```python
from build123d import *

# Parameters (mm, degrees)
F7_DEPTH  = 355.6
F8_D      = 12.7
F8_DEPTH  = 19.051
F9_D      = 12.7
F0_R      = 4.7625
F2_DEPTH  = 4.7625
F4_D      = 9.525
F4_DEPTH  = 19.051
F5_D      = 12.7
F5_DEPTH  = 19.051
F10_D     = 22.225
F10_DEPTH = 19.051
F6_DEPTH  = 25.4


with BuildPart() as f7:
    # F0 (on Front) → F7 (new body)
    with BuildSketch(Plane.XZ):
        with BuildLine():
            Line((-15.875, -19.05), (15.875, -19.05))
            ThreePointArc((15.875, -19.05), (18.1200640303, -18.1200640303), (19.05, -15.875))
            Line((19.05, -15.875), (19.05, 15.875))
            ThreePointArc((19.05, 15.875), (18.1200640303, 18.1200640303), (15.875, 19.05))
            Line((15.875, 19.05), (-15.875, 19.05))
            ThreePointArc((-15.875, 19.05), (-18.1200640303, 18.1200640303), (-19.05, 15.875))
            Line((-19.05, 15.875), (-19.05, -15.875))
            ThreePointArc((-19.05, -15.875), (-18.1200640303, -18.1200640303), (-15.875, -19.05))
        make_face()
        with BuildLine():
            ThreePointArc((14.2875, -11.1125), (13.3575640303, -13.3575640303), (11.1125, -14.2875))
            Line((11.1125, -14.2875), (-11.1125, -14.2875))
            ThreePointArc((-11.1125, -14.2875), (-13.3575640303, -13.3575640303), (-14.2875, -11.1125))
            Line((-14.2875, -11.1125), (-14.2875, 11.1125))
            ThreePointArc((-14.2875, 11.1125), (-13.3575640303, 13.3575640303), (-11.1125, 14.2875))
            Line((-11.1125, 14.2875), (11.1125, 14.2875))
            ThreePointArc((11.1125, 14.2875), (13.3575640303, 13.3575640303), (14.2875, 11.1125))
            Line((14.2875, 11.1125), (14.2875, -11.1125))
        make_face(mode=Mode.SUBTRACT)
    extrude(amount=F7_DEPTH)

    # F8 (through all, one way)
    with BuildSketch(Plane.XY):
        with Locations((0, -19.05)):
            Circle(F8_D / 2)
    extrude(amount=-F8_DEPTH, mode=Mode.SUBTRACT)

    # F9 (through all)
    with Locations(Plane(origin=(0, 0, 0), x_dir=(1, 0, 0), z_dir=(0, 0, -1))):
        with Locations((0, 19.05)):
            Hole(F9_D / 2)

    # F0 (on Front) → F2 (join)
    with BuildSketch(Plane.XZ):
        with BuildLine():
            Line((-11.1125, -14.2875), (11.1125, -14.2875))
            ThreePointArc((11.1125, -14.2875), (13.3575640303, -13.3575640303), (14.2875, -11.1125))
            Line((14.2875, -11.1125), (14.2875, 11.1125))
            ThreePointArc((14.2875, 11.1125), (13.3575640303, 13.3575640303), (11.1125, 14.2875))
            Line((11.1125, 14.2875), (-11.1125, 14.2875))
            ThreePointArc((-11.1125, 14.2875), (-13.3575640303, 13.3575640303), (-14.2875, 11.1125))
            Line((-14.2875, 11.1125), (-14.2875, -11.1125))
            ThreePointArc((-14.2875, -11.1125), (-13.3575640303, -13.3575640303), (-11.1125, -14.2875))
        make_face()
        Circle(F0_R, mode=Mode.SUBTRACT)
        Circle(F0_R)
    extrude(amount=F2_DEPTH)

    # F4 (through all, one way)
    with BuildSketch(Plane(origin=(0, 0, 0), x_dir=(0, 1, 0), z_dir=(-1, 0, 0))):
        with Locations((-50.8, 0)):
            Circle(F4_D / 2)
    extrude(amount=-F4_DEPTH, mode=Mode.SUBTRACT)

    # F5 (through all, one way)
    with BuildSketch(Plane.YZ):
        with Locations((-50.8, 0)):
            Circle(F5_D / 2)
    extrude(amount=-F5_DEPTH, mode=Mode.SUBTRACT)

    # F10 (through all, one way)
    with BuildSketch(Plane.YZ):
        with Locations((-82.55, 0)):
            Circle(F10_D / 2)
    extrude(amount=-F10_DEPTH, mode=Mode.SUBTRACT)

    # F0 (on Front) → F6 (join)
    with BuildSketch(Plane.XZ):
        Circle(F0_R)
    extrude(amount=-F6_DEPTH)


solid = f7.part
```
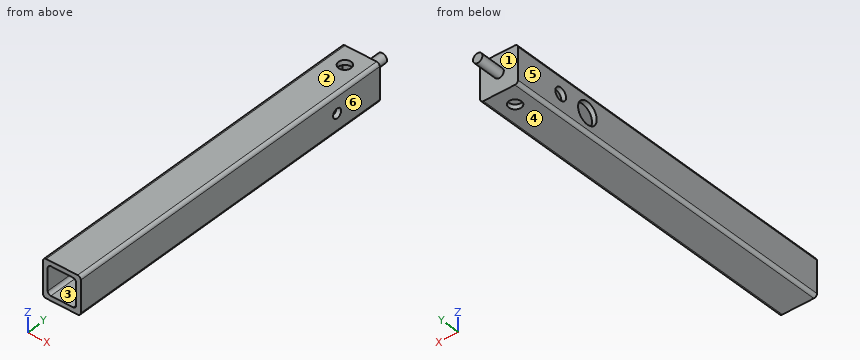
Design review of the part built by this model. Coordinates are the model's own, in mm. Face numbers are marked on the shaded views. A direction names the side the tool comes from. Coordinates: 2 decimals unless noted, no trailing zeros. Order: outer loops, then holes, each group sorted by start corner. A loop starts at its lowest first (then second) coordinate and runs counter-clockwise, first axis right, second up. Notation, with made-up numbers: (84, -25.75) - (98, -25.75) arc R31 ccw to (98, 10.25) - close; hole circle Ø1 at (89.5, 21.25). An arc over 180 degrees is marked (long way). Answer in a Markdown table with one row per item.
(1) The part is to be moulded in two halves that separate along X. For the marked faces 3, 4, 5 and 6, say which applies: released by +X, released by -X, zero draft, split by the parting line, or undercut.
Checked values:
| item | result |
|---|---|
| face 3 | undercut |
| face 4 | zero draft |
| face 5 | released by -X |
| face 6 | released by +X |
(2) Clearance check with flat-ended pins moving along their axes: pin 1 (1.5 mm diameter, centred on x = 9, z = 4.5, fed in from -Y); pin 2 (14.5 mm diameter, centred on y = -50.8, z = 0, fed in from +X); pin 3 (18 mm diameter, centred on y = -82.55, z = 0, fed in from -X). State where each tip first meets the part, or that it passes through.
Checked values:
| item | result |
|---|---|
| pin 1 | y = -4.76 |
| pin 2 | x = 19.05 |
| pin 3 | x = 14.29 |
(3) For the marked faces 1 and 2, list the 3-axis set-ups (+Z, -Z, +X, -X, +Y, -Y) from which the entire face can be reached by the end or side of a thin tool; tool diameter is ignored.
Checked values:
| item | result |
|---|---|
| face 1 | +Y |
| face 2 | +Z, +X, -X, +Y, -Y |
(4) Consider section B-B on x = 0. State the section outline as (y, z) points, plus the area to 3 significant figures.
Checked values:
| item | result |
|---|---|
| outline | (-355.6, -19.05) - (-25.4, -19.05) - (-25.4, -14.29) - (-355.6, -14.29) - close; (-355.6, 14.29) - (-25.4, 14.29) - (-25.4, 19.05) - (-355.6, 19.05) - close; (-12.7, -19.05) - (0, -19.05) - (0, -4.76) - (25.4, -4.76) - (25.4, 4.76) - (0, 4.76) - (0, 19.05) - (-12.7, 19.05) - (-12.7, 14.29) - (-4.76, 14.29) - (-4.76, -14.29) - (-12.7, -14.29) - close |
| area | 3,640 mm^2 |
(5) Wall thickness on line 1 along X through (y, z) = (-244.5, -11); line 2 along Z through (x, y) = (11.5, -218.5); line 3 along Y through (x, z) = (0, 16.8): over which ranges is each line inside the solid? List them lowest first. Write a range as from..to.
Checked values:
| item | result |
|---|---|
| line 1 | -19.05..-14.29, 14.29..19.05 |
| line 2 | -19.05..-14.26, 14.26..19.05 |
| line 3 | -355.6..-25.4, -12.7..0 |
